Here's how the part is built. I have some questions about the finished solid (model axes, mm). Coordinates: 2 decimals unless noted, no trailing zeros. Write each loop counter-clockwise with the first axis right and the second up, starting at its lowest first coordinate (ties: lowest second). Pieces come first, ordered by that corner, then holes. Notation, with made-up numbers: (60.5, 5) - (69.5, 5) arc R24 ccw to (69.5, 20) - close; hole circle Ø9 at (-4, 37.5). An arc over 180 degrees is marked (long way). Answer in a Markdown table with one row per item. Add a question column.
Item 1: We'd pull the mould along Z, two halves only. Please class faces 1 (the face through (0, 0, 0)), 2 (the face through (-15, 0, 5)), 3 (the face through (2, 0, 3)), 4 (the face through (-17.535, 0.429, 5.306)): +Z half, -Z half, draft (parallel to the pull), parting line (faces both ways), or undercut.
Item 2: I'm going to push flat-ended pins straight in: pin 1 (12 mm diameter, centred on x = -3.5, y = -5, fed in from +Z); pin 2 (4 mm diameter, centred on x = 6.5, y = -5, fed in from -Z); pin 3 (10 mm diameter, centred on x = -8.5, z = 13.5, fed in from -Y); pin 4 (4 mm diameter, centred on x = -15, y = -9.5, fed in from +Z). Where does each tip first touch, or does it pass through?
Item 3: Imagine slicing it at C-C (z = 9). Please give me the cut outline in (x, y), plus the area to 3 significant figures.
Item 4: Imagine slicing it at A-A (z = 17). Please give me the cut outline in (x, y), plus the area to 3 significant figures.
Item 5: If I drill on probe 1 along X at (y, z) = (12, 6.75); probe 2 along Z at (x, y) = (2, -8); probe 3 along Z at (x, y) = (-16.45, 0), over which ranges is the centre line in solid material (lowest first)? Write a range as from..to.
Item 6: Imagine slicing it at D-D (x = 1.5). Please give me the cut outline in (y, z).
Item 7: Imagine slicing it at B-B (y = 15). Please give me the cut outline in (x, z), plus the area to 3 significant figures.
from build123d import *

# Parameters (mm, degrees)
F0_W     = 40
F0_H     = 35
F1_DEPTH = 3
F2_R     = 5
F3_W     = 5
F3_H     = 35
F4_DEPTH = 40
F6_DEPTH = 40.001


with BuildPart() as f1:
    # F0 (on Top) → F1 (new body)
    with BuildSketch(Plane.XY):
        Rectangle(F0_W, F0_H)
    extrude(amount=F1_DEPTH)

    # F2
    f2_edges = [f1.edges().sort_by_distance(p)[0] for p in [
        (20, 17.5, 1.5),
        (20, -17.5, 1.5),
    ]]
    fillet(f2_edges, radius=F2_R)

    # F3 (on face) → F4 (join)
    with BuildSketch(Plane.XY.offset(3)):
        with Locations((-17.5, 0)):
            Rectangle(F3_W, F3_H)
    extrude(amount=F4_DEPTH)

    # F5 (on face) → F6 (cut, through all)
    with BuildSketch(Plane(origin=(-20, 0, 0), x_dir=(0, -1, 0), z_dir=(-1, 0, 0))):
        with BuildLine():
            Line((-17.5, 26.898632), (-14.25, 26.898632))
            ThreePointArc((-14.25, 26.898632), (0, 5.300476), (14.25, 26.898632))
            Line((14.25, 26.898632), (17.5, 26.898632))
            Line((17.5, 26.898632), (17.5, 43))
            Line((17.5, 43), (-17.5, 43))
            Line((-17.5, 43), (-17.5, 26.898632))
        make_face()
    extrude(amount=-F6_DEPTH, mode=Mode.SUBTRACT)


solid = f1.part
Here are the results:
| question | item | result |
|---|---|---|
| 1 | face 1 | -Z half |
| 1 | face 2 | draft |
| 1 | face 3 | +Z half |
| 1 | face 4 | undercut |
| 2 | pin 1 | stops at z = 3 |
| 2 | pin 2 | stops at z = 0 |
| 2 | pin 3 | passes through |
| 2 | pin 4 | stops at z = 10.41 |
| 3 | outline | (-20, -17.5) - (-15, -17.5) - (-15, -10.05) - (-20, -10.05) - close; (-20, 10.05) - (-15, 10.05) - (-15, 17.5) - (-20, 17.5) - close |
| 3 | area | 74.5 mm2 |
| 4 | outline | (-20, -17.5) - (-15, -17.5) - (-15, -15.03) - (-20, -15.03) - close; (-20, 15.03) - (-15, 15.03) - (-15, 17.5) - (-20, 17.5) - close |
| 4 | area | 24.7 mm2 |
| 5 | probe 1 | x = -20..-15 |
| 5 | probe 2 | z = 0..3 |
| 5 | probe 3 | z = 0..5.3 |
| 6 | outline | (-17.5, 0) - (17.5, 0) - (17.5, 3) - (-17.5, 3) - close |
| 7 | outline | (-20, 0) - (19.33, 0) - (19.33, 3) - (-15, 3) - (-15, 16.9) - (-20, 16.9) - close; (-20, 24.71) - (-15, 24.71) - (-15, 26.9) - (-20, 26.9) - close |
| 7 | area | 198 mm2 |
